```python
from build123d import *

# Parameters (mm, degrees)
SKETCH1_R           = 45
BOSS_EXTRUDE1_DEPTH = 80
BOSS_EXTRUDE2_REACH = 112
SKETCH2_W           = 63
SKETCH2_H           = 80
FILLET1_R           = 5
SKETCH3_R           = 5
BOSS_EXTRUDE3_DEPTH = 10
SKETCH4_W           = 147
SKETCH4_H           = 147
BOSS_EXTRUDE4_DEPTH = 4
SKETCH5_R           = 2.5
CUT_EXTRUDE1_DEPTH  = 5
FILLET2_R           = 8


with BuildPart() as part:
    # Sketch1 → Boss-Extrude1 (new body)
    with BuildSketch(Plane(origin=(0, 0, 0), x_dir=(1, 0, 0), z_dir=(0, 1, 0))):
        Circle(SKETCH1_R)
    extrude(amount=BOSS_EXTRUDE1_DEPTH)

    # Sketch2 → Boss-Extrude2 (add, up to next)
    with BuildSketch(Plane(origin=(65, 0, 0), x_dir=(0, 0, -1), z_dir=(1, 0, 0)), mode=Mode.PRIVATE) as boss_extrude2_sk1:
        with Locations((0, 40)):
            Rectangle(SKETCH2_W, SKETCH2_H)
    boss_extrude2_tool1 = extrude(boss_extrude2_sk1.sketch, amount=-BOSS_EXTRUDE2_REACH, mode=Mode.PRIVATE) - part.part
    add(boss_extrude2_tool1.solids().sort_by_distance((65, 40, 0))[0])

    # Fillet1
    fillet1_edges = [part.edges().sort_by_distance(p)[0] for p in [
        (-45, 80, 0),
        (32.136427928, 40, -31.5),
        (48.568213964, 80, -31.5),
        (48.568213964, 80, 31.5),
        (32.136427928, 40, 31.5),
    ]]
    fillet(fillet1_edges, radius=FILLET1_R)

    # Sketch3 → Boss-Extrude3 (add)
    with BuildSketch(Plane(origin=(0, 80, 0), x_dir=(1, 0, 0), z_dir=(0, 1, 0))):
        Circle(SKETCH3_R)
    extrude(amount=BOSS_EXTRUDE3_DEPTH)

    # Sketch4 → Boss-Extrude4 (add)
    with BuildSketch(Plane.XZ):
        with Locations((10, 0)):
            Rectangle(SKETCH4_W, SKETCH4_H)
    extrude(amount=BOSS_EXTRUDE4_DEPTH)

    # Sketch5 → Cut-Extrude1 (cut, through all)
    with BuildSketch(Plane(origin=(0, 0, 0), x_dir=(1, 0, 0), z_dir=(0, 1, 0))):
        with Locations((-53.5, 63.5)):
            Circle(SKETCH5_R)
        with Locations((73.5, 63.5)):
            Circle(SKETCH5_R)
        with Locations((-53.5, -63.5)):
            Circle(SKETCH5_R)
        with Locations((73.5, -63.5)):
            Circle(SKETCH5_R)
    extrude(amount=-CUT_EXTRUDE1_DEPTH, mode=Mode.SUBTRACT)

    # Fillet2
    fillet2_edges = [part.edges().sort_by_distance(p)[0] for p in [
        (-63.5, -2, 73.5),
        (-63.5, -2, -73.5),
        (83.5, -2, -73.5),
        (83.5, -2, 73.5),
    ]]
    fillet(fillet2_edges, radius=FILLET2_R)


solid = part.part
```
Verification items for the finished model (mm, model axes). A direction names the side the tool comes from. Round coordinates to 2 decimals unless told otherwise and drop trailing zeros. Write each loop counter-clockwise with the first axis right and the second up, starting at its lowest first coordinate (ties: lowest second). Pieces come first, ordered by that corner, then holes. Notation, with made-up numbers: (80, 23.25) - (95, 23.25) arc R18 ccw to (95, 55.25) - close; hole circle Ø7 at (-23, 54.5). An arc over 180 degrees is marked (long way). Answer as a JSON object with one key per item and string values. Group by question number.
Q1. Section check A-A, the plane x = 73.5. Enter the section's corners in (y, z).
Q2. Section check B-B, the plane z = 63.5. Enter the section's corners in (x, y), plus the area to 3 significant figures.
Q3. Tool access check on faces 5 (the flat face through (65, 41, 0)), 6 (the flat face through (9, -2, 73.5)), 7 (the flat face through (50, 37, 31.5)), 8 (the flat face through (50, 37, -31.5)), 9 (the cylindrical face through (-1.08, 84.93, 4.88)). Record the directions out of +Z, -Z, +X, -X, +Y, -Y that give a thin tool (end or side, any length) a straight path to the whole face; none if there is none.
Q4. Mould release check, pull along X, two halves, no side actions. Record for faces 1 (the flat face through (83.5, -2, -1)), 2 (the cylindrical face through (-51.19, -1.97, 64.46)), 3 (the flat face through (0, 90, 0)), 4 (the cylindrical face through (-61.219, -2.028, 71.094)): released by +X, released by -X, zero draft, split by the parting line, or undercut.
Q5. Thickness scan on line 1 (X direction, y = -1.65, z = 63.5); line 2 (Z direction, x = 73.5, y = -2); line 3 (X direction, y = -2, z = 63). Record the ranges inside material, lowest first.
Q6. Section check C-C, the plane y = 9. Enter the section's corners in (x, z), plus the area to 3 significant figures.
Q7. Go/stop test with flat-tipped pins: pin 1 Ø6 at (x, z) = (-53.5, 63.5) entering from -Y; pin 2 Ø8 at (x, z) = (73.5, -63.5) entering from +Y; pin 3 Ø3 at (y, z) = (11, -25.5) entering from +X; pin 4 Ø3 at (x, z) = (33.5, 14.5) entering from +Y. Record where each tip stops, or that it passes through.
Q8. Section check D-D, the plane z = 0. Enter the section's corners in (x, y), plus the area to 3 significant figures.
Found:
{
 "1": {"outline": "(-4, -73.5) - (0, -73.5) - (0, -66) - (-4, -66) - close; (-4, -61) - (0, -61) - (0, 61) - (-4, 61) - close; (-4, 66) - (0, 66) - (0, 73.5) - (-4, 73.5) - close"},
 "2": {"outline": "(-63.5, -4) - (-56, -4) - (-56, 0) - (-63.5, 0) - close; (-51, -4) - (71, -4) - (71, 0) - (-51, 0) - close; (76, -4) - (83.5, -4) - (83.5, 0) - (76, 0) - close", "area": "548 mm^2"},
 "3": {"face 5": "+Z, -Z, +X, +Y", "face 6": "+Z, +X, -X, +Y, -Y", "face 7": "+Z, +X, +Y", "face 8": "-Z, +X, +Y", "face 9": "+Y"},
 "4": {"face 1": "released by +X", "face 2": "undercut", "face 3": "zero draft", "face 4": "released by -X"},
 "5": {"line 1": "x = -63.5 to -56, -51 to 71, 76 to 83.5", "line 2": "z = -73.5 to -66, -61 to 61, 66 to 73.5", "line 3": "x = -63.5 to -55.95, -51.05 to 71.05, 75.95 to 83.5"},
 "6": {"outline": "(30.76, -32.85) arc R5 cw to (34.17, -31.5) - (65, -31.5) - (65, 31.5) - (34.17, 31.5) arc R5 cw to (30.76, 32.85) arc R45 ccw (long way) to start", "area": "7,880 mm^2"},
 "7": {"pin 1": "stops at y = -4", "pin 2": "stops at y = 0", "pin 3": "stops at x = 65", "pin 4": "stops at y = 80"},
 "8": {"outline": "(-63.5, -4) - (83.5, -4) - (83.5, 0) - (65, 0) - (65, 80) - (5, 80) - (5, 90) - (-5, 90) - (-5, 80) - (-40, 80) arc R5 ccw to (-45, 75) - (-45, 0) - (-63.5, 0) - close", "area": "9,480 mm^2"}
}
